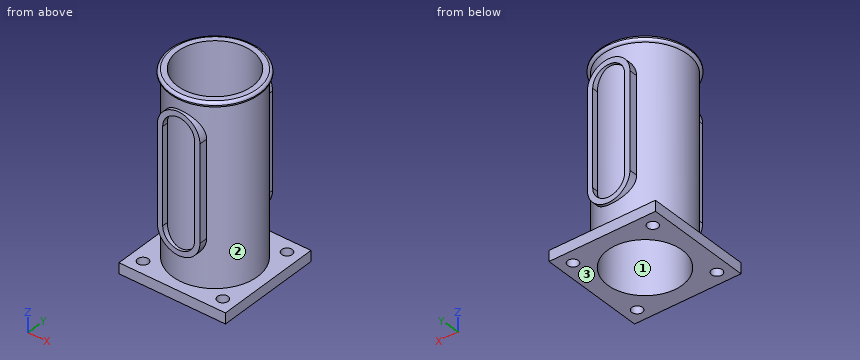
```python
from build123d import *

# Parameters (mm, degrees)
SKETCH2_W                     = 63.5
SKETCH2_H                     = 63.5
SKETCH2_R                     = 22.225
BOSS_EXTRUDE1_DEPTH           = 6.35
SKETCH3_R                     = 25.4
SKETCH3_R_2                   = 22.225
BOSS_EXTRUDE2_DEPTH           = 101.6
SKETCH4_W                     = 63.5
SKETCH4_H                     = 63.5
SKETCH4_R                     = 22.225
BOSS_EXTRUDE3_DEPTH           = 6.35
F_3_0_25_DIAMETER_HOLE1_D     = 6.35
F_3_0_25_DIAMETER_HOLE1_DEPTH = 6.35
SKETCH8_W                     = 63.5
SKETCH8_H                     = 63.5
CUT_EXTRUDE1_DEPTH            = 3.175
BOSS_EXTRUDE4_REACH           = 118.916
SKETCH9_R                     = 25.4
SKETCH9_R_2                   = 22.225
SKETCH10_OUTSIDE_W            = 94.572
SKETCH10_OUTSIDE_H            = 94.572
SKETCH10_OUTSIDE_R            = 26.9875
CUT_EXTRUDE2_DEPTH            = 3.175
FILLET1_R                     = 1.5875
BOSS_EXTRUDE5_DEPTH           = 26.9875
CUT_EXTRUDE3_DEPTH            = 123.80315559
CUT_EXTRUDE3_DEPTH_BACK       = 123.80315559
SKETCH12_R                    = 22.225


with BuildPart() as part:
    # Sketch2 → Boss-Extrude1 (new body)
    with BuildSketch(Plane.XY):
        Rectangle(SKETCH2_W, SKETCH2_H)
        Circle(SKETCH2_R, mode=Mode.SUBTRACT)
    extrude(amount=BOSS_EXTRUDE1_DEPTH)

    # Sketch3 → Boss-Extrude2 (add)
    with BuildSketch(Plane.XY.offset(6.35)):
        with Locations(Location((0, 0, 0), (0, 0, 180))):
            Circle(SKETCH3_R)
        Circle(SKETCH3_R_2, mode=Mode.SUBTRACT)
    extrude(amount=BOSS_EXTRUDE2_DEPTH)

    # Sketch4 → Boss-Extrude3 (add)
    with BuildSketch(Plane.XY.offset(107.95)):
        Rectangle(SKETCH4_W, SKETCH4_H)
        Circle(SKETCH4_R, mode=Mode.SUBTRACT)
    extrude(amount=BOSS_EXTRUDE3_DEPTH)

    # #3 (0.25) Diameter Hole1
    with Locations(Plane(origin=(0, 0, 0), x_dir=(-1, 0, 0), z_dir=(0, 0, -1))):
        with Locations((-23.8125, 23.8125), (-23.8125, -23.8125), (23.8125, -23.8125), (23.8125, 23.8125)):
            Hole(F_3_0_25_DIAMETER_HOLE1_D / 2, depth=F_3_0_25_DIAMETER_HOLE1_DEPTH)

    # Sketch8 → Cut-Extrude1 (cut)
    with BuildSketch(Plane(origin=(0, 0, 107.95), x_dir=(-1, 0, 0), z_dir=(0, 0, -1))):
        Rectangle(SKETCH8_W, SKETCH8_H)
    extrude(amount=-CUT_EXTRUDE1_DEPTH, mode=Mode.SUBTRACT)


with BuildPart() as cut_extrude1_piece_1:
    # of the separate pieces the step leaves, piece 1, a body of its own (cut_extrude1_pieces)
    add(part.part.solids().sort_by_distance((-31.75, -31.75, 0))[0])


with BuildPart() as cut_extrude1_piece_2:
    # of the separate pieces the step leaves, piece 2, a body of its own (cut_extrude1_pieces)
    add(part.part.solids().sort_by_distance((22.225, 0, 111.125))[0])

    # Sketch9 → Boss-Extrude4 (add, up to next)
    with BuildSketch(Plane.XY.offset(107.95), mode=Mode.PRIVATE) as boss_extrude4_sk1:
        with Locations(Location((0, 0, 0), (0, 0, 180))):
            Circle(SKETCH9_R)
        Circle(SKETCH9_R_2, mode=Mode.SUBTRACT)
    boss_extrude4_tool1 = extrude(boss_extrude4_sk1.sketch, amount=BOSS_EXTRUDE4_REACH, mode=Mode.PRIVATE) - cut_extrude1_piece_2.part

    add(cut_extrude1_piece_1.part)  # Boss-Extrude4 merges Cut-Extrude1 piece 1
    add(boss_extrude4_tool1.solids().sort_by_distance((24.68158, 0, 107.95))[0])

    # Sketch10 outside → Cut-Extrude2 (cut)
    with BuildSketch(Plane.XY.offset(114.3)):
        Rectangle(SKETCH10_OUTSIDE_W, SKETCH10_OUTSIDE_H)
        Circle(SKETCH10_OUTSIDE_R, mode=Mode.SUBTRACT)
    extrude(amount=-CUT_EXTRUDE2_DEPTH, mode=Mode.SUBTRACT)

    # Fillet1
    fillet1_edges = [cut_extrude1_piece_2.edges().sort_by_distance(p)[0] for p in [
        (-26.9875, 0, 111.125),
        (-26.9875, 0, 114.3),
    ]]
    fillet(fillet1_edges, radius=FILLET1_R - 0.0001)  # a hair under: the kernel refuses the full size

    # Sketch11 → Boss-Extrude5 (add)
    with BuildSketch(Plane(origin=(0, 0, 0), x_dir=(1, 0, 0), z_dir=(0, 1, 0))):
        with BuildLine():
            Line((-12.7, -92.075), (-12.7, -34.925))
            ThreePointArc((-12.7, -34.925), (0, -22.225), (12.7, -34.925))
            Line((12.7, -34.925), (12.7, -92.075))
            ThreePointArc((12.7, -92.075), (0, -104.775), (-12.7, -92.075))
        make_face()
        with BuildLine():
            Line((-9.525, -92.075), (-9.525, -34.925))
            ThreePointArc((-9.525, -34.925), (0, -25.4), (9.525, -34.925))
            Line((9.525, -34.925), (9.525, -92.075))
            ThreePointArc((9.525, -92.075), (0, -101.6), (-9.525, -92.075))
        make_face(mode=Mode.SUBTRACT)
    boss_extrude5 = extrude(amount=BOSS_EXTRUDE5_DEPTH)

    # Mirror1: Boss-Extrude5 across plane
    add(boss_extrude5.mirror(Plane.ZX))

    # Sketch12 → Cut-Extrude3 (cut, two sides: drawn at the far end of the back side and taken through both)
    with BuildSketch(Plane(origin=(0, 0, 0), x_dir=(-1, 0, 0), z_dir=(0, 0, -1)).offset(-CUT_EXTRUDE3_DEPTH_BACK)):
        with Locations(Location((0, 0, 0), (0, 0, 180))):
            Circle(SKETCH12_R)
    extrude(amount=CUT_EXTRUDE3_DEPTH + CUT_EXTRUDE3_DEPTH_BACK, mode=Mode.SUBTRACT)


solid = cut_extrude1_piece_2.part
```
Here's how the part is built. I have some questions about the finished solid (model axes, mm). Face numbers are marked on the shaded views. Coordinates: 2 decimals unless noted, no trailing zeros. One line per item, written item: value.
1. Please list where these lines run through material, in increasing order: probe 1 along Z at (x, y) = (-20.5, 25.5); probe 2 along X at (y, z) = (18, 27); probe 3 along X at (y, z) = (-20, 75).
Geometry says:
probe 1: z = 0 to 6.35
probe 2: x = -17.92 to -13.04, 13.04 to 17.92
probe 3: x = -15.66 to -9.69, 9.69 to 15.66
2. Imagine slicing it at C-C (x = -24). State how many separate pieces and enclosed holes the cut face has, and give its area (3 significant figures).
Geometry says:
separate pieces: 3
enclosed holes: 0
area: 2,140 mm2
3. Will these pins go through, and if not, where does the flat tip stop? pin 1 Ø10 at (x, y) = (-23.81, 23.81) entering from +Z; pin 2 Ø5.5 at (x, y) = (23.81, 23.81) entering from -Z; pin 3 Ø1 at (x, z) = (19, 50) entering from -Y; pin 4 Ø4 at (y, z) = (-25, 63) entering from -X.
Geometry says:
pin 1: stops at z = 6.35
pin 2: passes through
pin 3: stops at y = -17.4
pin 4: stops at x = -12.7
4. Thinking about a two-plate mould opening in X: for the marked faces 1, 2 and 3, which applies, +X half, -X half, draft (parallel to the pull), parting line (faces both ways), or undercut?
Geometry says:
face 1: undercut
face 2: parting line
face 3: draft
